The model under review builds one solid part; all positions refer to its coordinate system, in mm. Round coordinates to 2 decimals unless told otherwise and drop trailing zeros. Write each loop counter-clockwise with the first axis right and the second up, starting at its lowest first coordinate (ties: lowest second). Pieces come first, ordered by that corner, then holes. Notation, with made-up numbers: (-7.75, 62) -> (6.25, 62) arc R20 cw to (6.25, 78) -> close; hole circle Ø7 at (11, 62.25). An arc over 180 degrees is marked (long way). Answer as a JSON object with one key per item and string values. Group by question number.
1) We need section D-D, the plane z = -30. Write out the cut boundary in (x, y), then the cut area to 3 significant figures.
2) We need section A-A, the plane y = 4.25. Write out the cut boundary in (x, z), then the cut area to 3 significant figures.
3) Mouldability with a two-part tool opening along X and no side actions: class faces 1 (the flat face through (11, 8, -75)), 2 (the flat face through (25, 14, 1)), 3 (the cylindrical face through (19.885, 12.874, 68.251)) as pulls with the +X half, pulls with the -X half, needs draft (parallel to the pull), parting line crosses it, or undercut.
4) We need section B-B, the plane x = -17.5. Write out the cut boundary in (y, z), then the cut area to 3 significant figures.
5) We need section C-C, the plane z = 67.5. Write out the cut boundary in (x, y).
6) To check wall thickness, follow probe 1 along Z at (x, y) = (17.5, 9); probe 2 along X at (y, z) = (3.45, -67.5); probe 3 along Z at (x, y) = (16, 7). State the ranges of each line that lie inside material, in increasing order. Write a range as [from, to].
7) Insertion check: pin 1 Ø6 at (y, z) = (10, -27) entering from -X; pin 2 Ø12 at (x, z) = (16, -10.5) entering from +Y; pin 3 Ø8 at (x, y) = (-10.5, 10) entering from -Z; pin 4 Ø5 at (x, z) = (4, -42.5) entering from +Y. Each pin has a flat end and moves straight along its axis. Give the tip position at first contact, or say it passes through.
from build123d import *

# Parameters (mm, degrees)
BOSS_EXTRUDE1_DEPTH = 75
SKETCH3_R           = 2.5
CUT_EXTRUDE1_DEPTH  = 50


with BuildPart() as part:
    # Sketch2 → Boss-Extrude1 (new body, symmetric)
    with BuildSketch(Plane.XY):
        Polygon((-25, 0), (25, 0), (25, 29), (-25, 0.132486541), align=None)
    extrude(amount=BOSS_EXTRUDE1_DEPTH, both=True)

    # Sketch3 → Cut-Extrude1 (cut)
    with BuildSketch(Plane.XZ):
        with Locations((-17.5, 67.5)):
            Circle(SKETCH3_R)
        with Locations((17.5, 67.5)):
            Circle(SKETCH3_R)
        with Locations((-17.5, -67.5)):
            Circle(SKETCH3_R)
        with Locations((17.5, -67.5)):
            Circle(SKETCH3_R)
    extrude(amount=-CUT_EXTRUDE1_DEPTH, mode=Mode.SUBTRACT)


solid = part.part
Here are the results:
{
 "1": {"outline": "(-25, 0) -> (25, 0) -> (25, 29) -> (-25, 0.13) -> close", "area": "728 mm^2"},
 "2": {"outline": "(-17.87, -75) -> (25, -75) -> (25, 75) -> (-17.87, 75) -> (-17.87, 69.97) arc R2.5 cw (long way) to (-17.87, 65.03) -> (-17.87, -65.03) arc R2.5 cw (long way) to (-17.87, -69.97) -> close; hole circle Ø5 at (17.5, -67.5); hole circle Ø5 at (17.5, 67.5)", "area": "6,370 mm^2"},
 "3": {"face 1": "needs draft", "face 2": "pulls with the +X half", "face 3": "undercut"},
 "4": {"outline": "(0, -75) -> (4.46, -75) -> (4.46, -70) -> (0, -70) -> close; (0, -65) -> (4.46, -65) -> (4.46, 65) -> (0, 65) -> close; (0, 70) -> (4.46, 70) -> (4.46, 75) -> (0, 75) -> close", "area": "625 mm^2"},
 "5": {"outline": "(-25, 0) -> (-20, 0) -> (-20, 3.02) -> (-25, 0.13) -> close; (-15, 0) -> (15, 0) -> (15, 23.23) -> (-15, 5.91) -> close; (20, 0) -> (25, 0) -> (25, 29) -> (20, 26.11) -> close"},
 "6": {"probe 1": "z = [-75, -70], [-65, 65], [70, 75]", "probe 2": "x = [-15, 15], [20, 25]", "probe 3": "z = [-75, -69.5], [-65.5, 65.5], [69.5, 75]"},
 "7": {"pin 1": "stops at x = -13.11", "pin 2": "stops at y = 27.27", "pin 3": "stops at z = -75", "pin 4": "stops at y = 18.32"}
}
